Read the model definition and answer for the solid it produces. Units are mm, in the model's axes. A direction names the side the tool comes from. Coordinates: 2 decimals unless noted, no trailing zeros. Write each loop counter-clockwise with the first axis right and the second up, starting at its lowest first coordinate (ties: lowest second). Pieces come first, ordered by that corner, then holes.
(1) Section B-B on z = -3.75 is taken. Write down the section's boundary in (x, y), then the cut area to 3 significant figures.
(2) Section A-A on x = 0 is taken. Write down the section's boundary in (y, z), then the cut area to 3 significant figures.
(3) Given pin 1 (8 mm diameter, centred on x = -15, y = 21.5, fed in from -Z); pin 2 (8 mm diameter, centred on y = 20.5, z = -10, fed in from -X); pin 3 (6 mm diameter, centred on x = 16.5, y = 8, fed in from -Z); pin 4 (1 mm diameter, centred on x = -19, z = -0.5, fed in from +Y), each flat-ended and moving along its own axis, determine where each tip first touches the part or whether it passes through.
(4) Section D-D on x = -6.5 is taken. Write down the section's boundary in (y, z).
(5) Which of the six approach directions +Z, -Z, +X, -X, +Y, -Y give full straight-line access (tool end or side, diameter ignored) to faces 1 (the flat face through (-18, 4, 0)), 2 (the flat face through (0, 27, 7)), 3 (the cylindrical face through (0.45, 27.01, 1.43)), 4 (the flat face through (19, 8, -5))?
(6) Find the intervals of material crossed by probe 1 along X at (y, z) = (0.95, 0); probe 2 along Y at (x, z) = (-3, -4); probe 3 along X at (y, z) = (6, -3.75), in increasing order.
(7) Section C-C on z = 0 is taken. Write down the section's boundary in (x, y).
(8) The mould has two halves that part along X. Classify faces 5 (the flat face through (0, 2, -1)), 6 (the flat face through (-7.5, 18, -12)), 7 (the flat face through (-1.4, 1.6, 10)): +X half, -X half, draft (parallel to the pull), parting line (faces both ways), or undercut.
from build123d import *

# Parameters (mm, degrees)
EXTRUDE_1_DEPTH     = 2
SKETCH_2_W          = 15
SKETCH_2_H          = 28
EXTRUDE_2_DEPTH     = 2
EXTRUDE_3_DEPTH     = 2
SKETCH_4_W          = 15
SKETCH_4_H          = 20
EXTRUDE_4_DEPTH     = 2
CUT_EXTRUDE_1_REACH = 37.285
SKETCH_5_R          = 1.6
CUT_EXTRUDE_2_REACH = 38.783
SKETCH_6_R          = 1.5


with BuildPart() as part:
    # 草图1 → 凸台-拉伸1 (new body)
    with BuildSketch(Plane(origin=(0, 0, 0), x_dir=(1, 0, 0), z_dir=(0, 1, 0))):
        Polygon((7.5, 10), (20, 10), (20, -10), (-20, -10), (-20, 10), (-7.5, 10), (-7.5, 13), (7.5, 13), align=None)
    extrude(amount=EXTRUDE_1_DEPTH)

    # 草图2 → 凸台-拉伸2 (add)
    with BuildSketch(Plane(origin=(0, 0, -13), x_dir=(-1, 0, 0), z_dir=(0, 0, -1))):
        with Locations((0, 14)):
            Rectangle(SKETCH_2_W, SKETCH_2_H)
    extrude(amount=-EXTRUDE_2_DEPTH)

    # 草图3 → 凸台-拉伸3 (add)
    with BuildSketch(Plane.ZY.offset(20)):
        Polygon((1.5, 4.5), (9, 12), (10, 12), (10, 0), (-10, 0), (-10, 12), (-9, 12), (-1.5, 4.5), align=None)
    extrude_3 = extrude(amount=-EXTRUDE_3_DEPTH)

    # 镜向1: 凸台-拉伸3 across plane
    add(extrude_3.mirror(Plane(origin=(0, 0, 0), x_dir=(0, 0, 1), z_dir=(1, 0, 0))))

    # 草图4 → 凸台-拉伸4 (add)
    with BuildSketch(Plane(origin=(0, 28, 0), x_dir=(1, 0, 0), z_dir=(0, 1, 0))):
        with Locations((0, 3)):
            Rectangle(SKETCH_4_W, SKETCH_4_H)
    extrude(amount=-EXTRUDE_4_DEPTH)

    # 草图5 → 切除-拉伸1 (cut, up to next)
    with BuildSketch(Plane(origin=(0, 2, 0), x_dir=(1, 0, 0), z_dir=(0, 1, 0)), mode=Mode.PRIVATE) as cut_extrude_1_sk1:
        with Locations(Location((-15, 0, 0), (0, 0, 270))):
            Circle(SKETCH_5_R)
    cut_extrude_1_tool1 = extrude(cut_extrude_1_sk1.sketch, amount=-CUT_EXTRUDE_1_REACH, mode=Mode.PRIVATE) & part.part
    # 草图5 → 切除-拉伸1 (cut, up to next)
    with BuildSketch(Plane(origin=(0, 2, 0), x_dir=(1, 0, 0), z_dir=(0, 1, 0)), mode=Mode.PRIVATE) as cut_extrude_1_sk2:
        with Locations(Location((15, 0, 0), (0, 0, 270))):
            Circle(SKETCH_5_R)
    cut_extrude_1_tool2 = extrude(cut_extrude_1_sk2.sketch, amount=-CUT_EXTRUDE_1_REACH, mode=Mode.PRIVATE) & part.part
    add(cut_extrude_1_tool1.solids().sort_by_distance((-15, 2, 0))[0], mode=Mode.SUBTRACT)
    add(cut_extrude_1_tool2.solids().sort_by_distance((15, 2, 0))[0], mode=Mode.SUBTRACT)

    # 草图6 → 切除-拉伸2 (cut, up to next)
    with BuildSketch(Plane(origin=(0, 28, 0), x_dir=(1, 0, 0), z_dir=(0, 1, 0)), mode=Mode.PRIVATE) as cut_extrude_2_sk1:
        with Locations(Location((0, 0, 0), (0, 0, 270))):
            Circle(SKETCH_6_R)
    cut_extrude_2_tool1 = extrude(cut_extrude_2_sk1.sketch, amount=-CUT_EXTRUDE_2_REACH, mode=Mode.PRIVATE) & part.part
    add(cut_extrude_2_tool1.solids().sort_by_distance((0, 28, 0))[0], mode=Mode.SUBTRACT)


solid = part.part
Response:
1. outline: (-20, 0) - (20, 0) - (20, 6.75) - (18, 6.75) - (18, 2) - (-18, 2) - (-18, 6.75) - (-20, 6.75) - close; (-7.5, 26) - (7.5, 26) - (7.5, 28) - (-7.5, 28) - close
1. area: 129 mm2
2. outline: (0, -13) - (28, -13) - (28, -1.5) - (26, -1.5) - (26, -11) - (2, -11) - (2, 10) - (0, 10) - close; (26, 1.5) - (28, 1.5) - (28, 7) - (26, 7) - close
2. area: 128 mm2
3. pin 1: passes through
3. pin 2: stops at x = -7.5
3. pin 3: stops at z = -10
3. pin 4: stops at y = 4.5
4. outline: (0, -13) - (28, -13) - (28, 7) - (26, 7) - (26, -11) - (2, -11) - (2, 10) - (0, 10) - close
5. face 1: +Z, -Z, +Y
5. face 2: +Z, +X, -X, +Y
5. face 3: +Y
5. face 4: +X, -X, +Y
6. probe 1: x = -20 to -16.6, -13.4 to 13.4, 16.6 to 20
6. probe 2: y = 0 to 2, 26 to 28
6. probe 3: x = -20 to -18, 18 to 20
7. outline: (-20, 0) - (-16.6, 0) - (-16.6, 2) - (-18, 2) - (-18, 4.5) - (-20, 4.5) - close; (-13.4, 0) - (13.4, 0) - (13.4, 2) - (-13.4, 2) - close; (-7.5, 26) - (-1.5, 26) - (-1.5, 28) - (-7.5, 28) - close; (1.5, 26) - (7.5, 26) - (7.5, 28) - (1.5, 28) - close; (16.6, 0) - (20, 0) - (20, 4.5) - (18, 4.5) - (18, 2) - (16.6, 2) - close
8. face 5: undercut
8. face 6: -X half
8. face 7: draft
